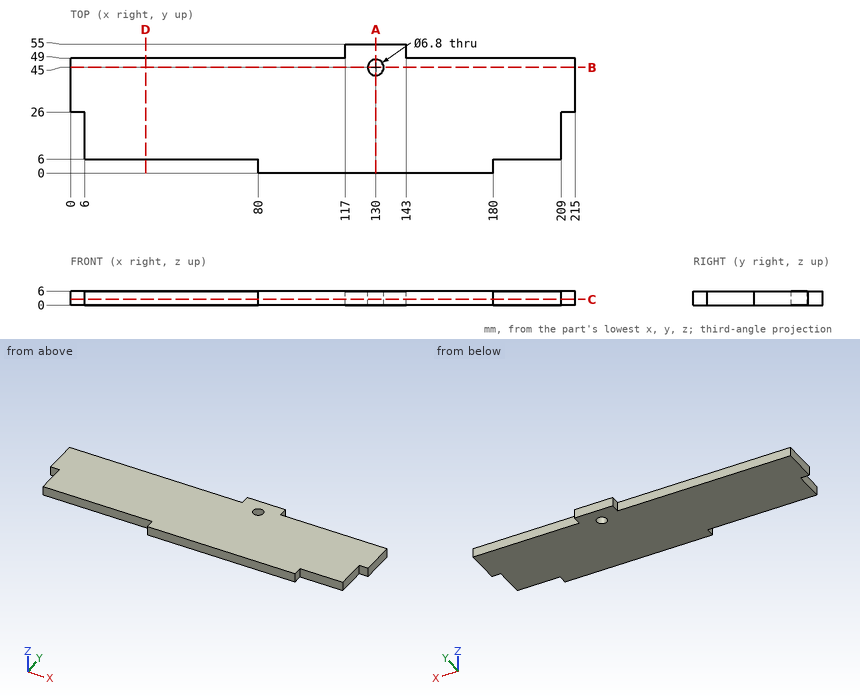
Input: dimensioned drawing with shaded views. Units: mm. Origin: part minimum x, y, z. Give positions to 0.01 mm unless a question says otherwise; leave off trailing zeros. Order: outer loops, then holes, each group sorted by start corner. A loop starts at its lowest first (then second) coordinate and runs counter-clockwise, first axis right, second up. Notation, with made-up numbers: (-15, 4.25) -> (15, 4.25) arc R23 ccw to (15, 12.25) -> close; hole circle Ø10 at (60, 16.5). An arc over 180 degrees is marked (long way). Answer as a JSON object with one key per item and string values.
Q1. Section C-C (z = 2.45). Output: boundary loops of the cut face in (x, y), plus the area to 3 significant figures.
Entries:
{"outline": "(0, 26) -> (6, 26) -> (6, 6) -> (80, 6) -> (80, 0) -> (180, 0) -> (180, 6) -> (209, 6) -> (209, 26) -> (215, 26) -> (215, 49) -> (143, 49) -> (143, 55) -> (117, 55) -> (117, 49) -> (0, 49) -> close; hole circle Ø6.8 at (130, 45)", "area": "9,720 mm^2"}
Q2. Section B-B (y = 45). Output: boundary loops of the cut face in (x, z).
Entries:
{"outline": "(0, 0) -> (126.6, 0) -> (126.6, 6) -> (0, 6) -> close; (133.4, 0) -> (215, 0) -> (215, 6) -> (133.4, 6) -> close"}
Q3. Material intervals for probe 1 along Y at (x, z) = (130, 4.3); probe 2 along Y at (x, z) = (70.5, 5.15); probe 3 along X at (y, z) = (23, 0.4), sorted ascending.
Entries:
{"probe 1": "y = 0 to 41.6, 48.4 to 55", "probe 2": "y = 6 to 49", "probe 3": "x = 6 to 209"}
Q4. Section D-D (x = 32). Output: boundary loops of the cut face in (y, z).
Entries:
{"outline": "(6, 0) -> (49, 0) -> (49, 6) -> (6, 6) -> close"}
Q5. Section A-A (x = 130). Output: boundary loops of the cut face in (y, z).
Entries:
{"outline": "(0, 0) -> (41.6, 0) -> (41.6, 6) -> (0, 6) -> close; (48.4, 0) -> (55, 0) -> (55, 6) -> (48.4, 6) -> close"}
Q6. First-contact query: pin 1 (1.8 mm diameter, centred on x = 195, z = 3.5, fed in from +Y); pin 2 (3 mm diameter, centred on x = 34.5, z = 5, fed in from -Y); pin 3 (1.8 mm diameter, centred on y = 17.5, z = 3, fed in from +X). Flat tips, straight axial feed; report the tip coordinate or a pass-through.
Entries:
{"pin 1": "stops at y = 49", "pin 2": "stops at y = 6", "pin 3": "stops at x = 209"}
